```python
from build123d import *

# Parameters (mm, degrees)
SKETCH1_W           = 200
SKETCH1_H           = 100
BOSS_EXTRUDE1_DEPTH = 5
SKETCH2_W           = 195
SKETCH2_H           = 95
BOSS_EXTRUDE2_DEPTH = 2.5
FILLET1_R           = 3
FILLET2_R           = 3


with BuildPart() as part:
    # Sketch1 → Boss-Extrude1 (new body)
    with BuildSketch(Plane(origin=(0, 0, 0), x_dir=(1, 0, 0), z_dir=(0, 1, 0))):
        with Locations((100, -50)):
            Rectangle(SKETCH1_W, SKETCH1_H)
    extrude(amount=BOSS_EXTRUDE1_DEPTH)

    # Sketch2 → Boss-Extrude2 (add)
    with BuildSketch(Plane(origin=(0, 5, 0), x_dir=(1, 0, 0), z_dir=(0, 1, 0))):
        with Locations((100, -50)):
            Rectangle(SKETCH2_W, SKETCH2_H)
    extrude(amount=BOSS_EXTRUDE2_DEPTH)

    # Fillet1
    fillet1_edges = [part.edges().sort_by_distance(p)[0] for p in [
        (0, 2.5, 0),
        (200, 2.5, 0),
        (200, 2.5, 100),
        (0, 2.5, 100),
    ]]
    fillet(fillet1_edges, radius=FILLET1_R)

    # Fillet2
    fillet2_edges = [part.edges().sort_by_distance(p)[0] for p in [
        (200, 0, 50),
        (0, 0, 50),
        (100, 0, 0),
        (100, 0, 100),
        (0.878679656, 0, 99.121320344),
        (0.878679656, 0, 0.878679656),
        (199.121320344, 0, 0.878679656),
        (199.121320344, 0, 99.121320344),
    ]]
    fillet(fillet2_edges, radius=FILLET2_R)


solid = part.part
```
CAD build for the part. Positions are in the model's coordinates, mm. Round coordinates to 2 decimals unless told otherwise and drop trailing zeros. Write each loop counter-clockwise with the first axis right and the second up, starting at its lowest first coordinate (ties: lowest second). Pieces come first, ordered by that corner, then holes. Notation, with made-up numbers: (-10, -24.5) - (24, -24.5) arc R26 ccw to (24, 10.5) - close; hole circle Ø3 at (-13.5, -19.75). An arc over 180 degrees is marked (long way). Return JSON: item names as keys, results as strings. Group by question number.
Item 1: Band-saw the part on B-B on y = 6.25. List the corners of the cut face in (x, z).
Item 2: Flat gauge pins, fed straight in: pin 1 Ø1.5 at (x, y) = (120.5, 6) entering from +Z; pin 2 Ø0.8 at (y, z) = (6, 37) entering from -X; pin 3 Ø2 at (y, z) = (6.5, 73.5) entering from +X. Where does each tip first touch, or does it go through?
Item 3: Mould opens along Y. For faces 1 (the face through (99, 7.5, 49)), 2 (the face through (99, 0, 49)) say: +Y half, -Y half, draft (parallel to the pull), parting line (faces both ways), or undercut.
Item 4: Probe probe 1 along Z at (x, y) = (94.5, 2.5); probe 2 along X at (y, z) = (5.25, 26); probe 3 along Z at (x, y) = (14.5, 7.25). List the from-to ranges inside material, lowest first.
Item 5: Band-saw the part on A-A on x = 136. List the corners of the cut face in (y, z).
Resolved:
{
 "1": {"outline": "(2.5, 2.5) - (197.5, 2.5) - (197.5, 97.5) - (2.5, 97.5) - close"},
 "2": {"pin 1": "stops at z = 97.5", "pin 2": "stops at x = 2.5", "pin 3": "stops at x = 197.5"},
 "3": {"face 1": "+Y half", "face 2": "-Y half"},
 "4": {"probe 1": "z = 0.04 to 99.96", "probe 2": "x = 2.5 to 197.5", "probe 3": "z = 2.5 to 97.5"},
 "5": {"outline": "(0, 3) arc R3 ccw to (3, 0) - (5, 0) - (5, 2.5) - (7.5, 2.5) - (7.5, 97.5) - (5, 97.5) - (5, 100) - (3, 100) arc R3 ccw to (0, 97) - close"}
}
